CAD build for the part. Positions are in the model's coordinates, mm. Face numbers are marked on the shaded views. A direction names the side the tool comes from. Round coordinates to 2 decimals unless told otherwise and drop trailing zeros. Order: outer loops, then holes, each group sorted by start corner. A loop starts at its lowest first (then second) coordinate and runs counter-clockwise, first axis right, second up. Notation, with made-up numbers: M -21.75,49.5 L 29.25,49.5 A22 ccw 29.25,61.5 Z; hole C 76.5,11 d3. An arc over 180 degrees is marked long. Answer as a JSON object with one key per item and string values.
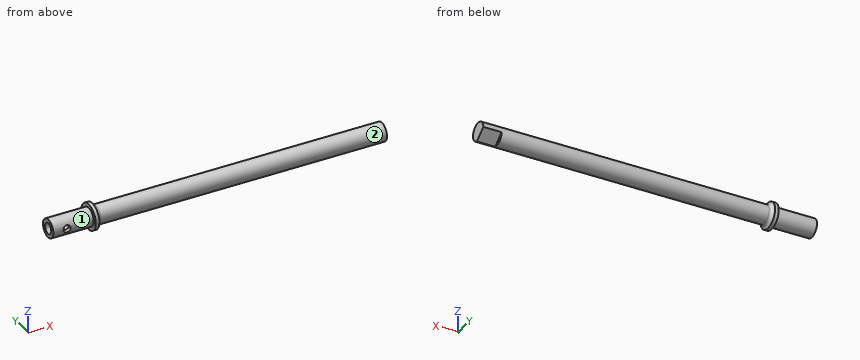
```python
from build123d import *

# Parameters (mm, degrees)
ESQUISSE1_W                  = 36
ESQUISSE1_H                  = 5
ESQUISSE1_W_2                = 2
ESQUISSE1_H_2                = 2
CONG_1_R                     = 2
ESQUISSE6_R                  = 2
ENL_V_MAT_EXTRU_2_DEPTH      = 5
ESQUISSE7_R                  = 3
ENL_V_MAT_EXTRU_3_DEPTH      = 16.3
ENL_V_MAT_EXTRU_4_DEPTH      = 183.269032028
ENL_V_MAT_EXTRU_4_DEPTH_BACK = 10


with BuildPart() as part:
    # Esquisse1 → Révolution1 (revolve)
    with BuildSketch(Plane.XY, mode=Mode.PRIVATE) as r_volution1_sk:
        Polygon((0, 5), (0, 0), (146, 0), (146, 5), (24, 5), (22, 5), align=None)
        with Locations((164, 2.5)):
            Rectangle(ESQUISSE1_W, ESQUISSE1_H)
        with Locations((23, 6)):
            Rectangle(ESQUISSE1_W_2, ESQUISSE1_H_2)
    revolve(r_volution1_sk.sketch.rotate(Axis((-22.396751432, 0, 0), (1, 0, 0)), 90), axis=Axis((-22.396751432, 0, 0), (1, 0, 0)))

    # Congé1
    cong_1_edges = [part.edges().sort_by_distance(p)[0] for p in [
        (24, 0, -5),
    ]]
    fillet(cong_1_edges, radius=CONG_1_R - 0.0001)  # a hair under: the kernel refuses the full size

    # Esquisse6 → Enlèv. mat.-Extru.2 (cut)
    with BuildSketch(Plane(origin=(0, -5, 0), x_dir=(-1, 0, 0), z_dir=(0, -1, 0))):
        with Locations(Location((-7.5, 0, 0), (0, 0, 180))):
            Circle(ESQUISSE6_R)
    extrude(amount=-ENL_V_MAT_EXTRU_2_DEPTH, mode=Mode.SUBTRACT)

    # Esquisse7 → Enlèv. mat.-Extru.3 (cut)
    with BuildSketch(Plane.ZY):
        Circle(ESQUISSE7_R)
    extrude(amount=-ENL_V_MAT_EXTRU_3_DEPTH, mode=Mode.SUBTRACT)

    # Esquisse8 → Enlèv. mat.-Extru.4 (cut, two sides: drawn at the far end of the back side and taken through both)
    with BuildSketch(Plane(origin=(182, 0, 0), x_dir=(0, 0, -1), z_dir=(1, 0, 0)).offset(-ENL_V_MAT_EXTRU_4_DEPTH_BACK)):
        Polygon((-23.820180397, 35.700913916), (0, 5), (4.843224662, -1.2422459), (28.663405059, -31.943159816), (90.065232892, 15.697200979), (37.581647435, 83.341274711), align=None)
    extrude(amount=ENL_V_MAT_EXTRU_4_DEPTH + ENL_V_MAT_EXTRU_4_DEPTH_BACK, mode=Mode.SUBTRACT)


solid = part.part
```
Item 1: Saw through at A-A on x = 72. List the corners of the cut face in (y, z).
Worked answers:
{"outline": "C 0,0 d10"}
Item 2: Wall check: line 1 along Y through (x, z) = (4.25, 0); line 2 along X through (y, z) = (-3.9, 0); line 3 along Z through (x, y) = (7.5, -3.4). Give the ranges that are in metal, low to high. Write a range as [from, to].
Worked answers:
{"line 1": "y = [-5, -3], [3, 5]", "line 2": "x = [0, 5.5], [9.5, 182]", "line 3": "z = [-3.67, -2], [2, 3.67]"}
Item 3: Saw through at B-B on x = 7.5. List the corners of the cut face in (y, z).
Worked answers:
{"outline": "M -4.58,-2 A5 ccw long -4.58,2 L -2.24,2 A3 cw long -2.24,-2 Z"}
Item 4: Drop flat-ended pins along their axis: pin 1 Ø6 at (x, z) = (111, -4) entering from +Y; pin 2 Ø2 at (x, y) = (101, 5.5) entering from +Z; pin 3 Ø1.8 at (y, z) = (-1, 1) entering from -X. Give the stop position or say it passes through.
Worked answers:
{"pin 1": "stops at y = 4.9", "pin 2": "stops at z = 2.18", "pin 3": "stops at x = 16.3"}
Item 5: 3-axis set-ups, long thin cutter, end or side, ignore diameter. For the marked faces 1 and 2: which of +Z, -Z, +X, -X, +Y, -Y reach the whole face in a straight line?
Worked answers:
{"face 1": "-X", "face 2": "+X"}
